from build123d import *

# Parameters (mm, degrees)
BOSS_EXTRUDE1_DEPTH = 148
FILLET1_R           = 1
SHELL1_T            = -1.5


with BuildPart() as part:
    # Sketch1 → Boss-Extrude1 (new body)
    with BuildSketch(Plane(origin=(0, 0, 0), x_dir=(1, 0, 0), z_dir=(0, 1, 0))):
        with BuildLine():
            Line((0, 0), (10.57, 0))
            Line((10.57, 0), (10.57, -30))
            Line((10.57, -30), (0, -30))
            ThreePointArc((0, -30), (2.434164903, -15), (0, 0))
        make_face()
    extrude(amount=BOSS_EXTRUDE1_DEPTH)

    # Fillet1
    fillet1_edges = [part.edges().sort_by_distance(p)[0] for p in [
        (10.57, 74, 0),
        (10.57, 74, 30),
    ]]
    fillet(fillet1_edges, radius=FILLET1_R)

    # Shell1
    shell1_openings = [part.faces().sort_by_distance(p)[0] for p in [
        (6.064557182, 148, 15),
        (6.064557182, 0, 15),
    ]]
    offset(amount=SHELL1_T, openings=shell1_openings, kind=Kind.INTERSECTION)


solid = part.part
Here's how the part is built. I have some questions about the finished solid (model axes, mm). A direction names the side the tool comes from. Round coordinates to 2 decimals unless told otherwise and drop trailing zeros. Order: outer loops, then holes, each group sorted by start corner. A loop starts at its lowest first (then second) coordinate and runs counter-clockwise, first axis right, second up. Notation, with made-up numbers: M 70,-34 L 111,-34 A17 cw 111,-28 Z; hole C 84,-5.5 d3. An arc over 180 degrees is marked long. Return JSON: item names as keys, results as strings. Group by question number.
1. If we section it at B-B on y = 53: List the corners of the cut face in (x, z) for me, then the cut area to 3 significant figures.
2. On a 3-axis mill with a long thin cutter (end or side, diameter ignored), from which of +Z, -Z, +X, -X, +Y, -Y can I reach the whole of each face in a straight line? I mean faces 5 (the face through (3.7, 0, 16)), 6 (the face through (6, 73, 28.5)). Say none if no direction works.
3. Please list where these lines run through material, in increasing order: probe 1 along Z at (x, y) = (8.5, 9.5); probe 2 along X at (y, z) = (28, 16.25); probe 3 along X at (y, z) = (17.5, 6.5).
4. If we section it at C-C on z = 2.75: List the corners of the cut face in (x, y) for me.
5. I'm going to push a flat-ended pin straight in: pin 1 Ø1.5 at (x, z) = (6, 13.5) entering from +Y. Where does the tip first touch, or does it pass through?
6. If we mould it in two halves opening along Z, with no side actions, what happens to faces 1 (the face through (5, 73, 0)), 2 (the face through (5, 73, 30)), 3 (the face through (2.434, 72.964, 15.214)), 4 (the face through (10.57, 73, 15))? For each: pulls with the +Z half, pulls with the -Z half, needs draft (parallel to the pull), parting line crosses it, or undercut.
7. If we section it at A-A on x = 7.25: List the corners of the cut face in (y, z) for me, then the cut area to 3 significant figures.
Reply:
{
 "1": {"outline": "M 0,0 L 9.57,0 A1 ccw 10.57,1 L 10.57,29 A1 ccw 9.57,30 L 0,30 A47.43 cw Z; hole M 2.04,1.5 L 9.07,1.5 L 9.07,28.5 L 2.04,28.5 A48.93 cw Z", "area": "112 mm^2"},
 "2": {"face 5": "+Z, -Z, +X, -X, -Y", "face 6": "+Y, -Y"},
 "3": {"probe 1": "0 to 1.5, 28.5 to 30", "probe 2": "2.42 to 3.92, 9.07 to 10.57", "probe 3": "1.67 to 3.19, 9.07 to 10.57"},
 "4": {"outline": "M 0.83,0 L 2.38,0 L 2.38,148 L 0.83,148 Z; M 9.07,0 L 10.57,0 L 10.57,148 L 9.07,148 Z"},
 "5": {"pin 1": "through"},
 "6": {"face 1": "pulls with the -Z half", "face 2": "pulls with the +Z half", "face 3": "undercut", "face 4": "needs draft"},
 "7": {"outline": "M 0,0 L 148,0 L 148,1.5 L 0,1.5 Z; M 0,28.5 L 148,28.5 L 148,30 L 0,30 Z", "area": "444 mm^2"}
}
